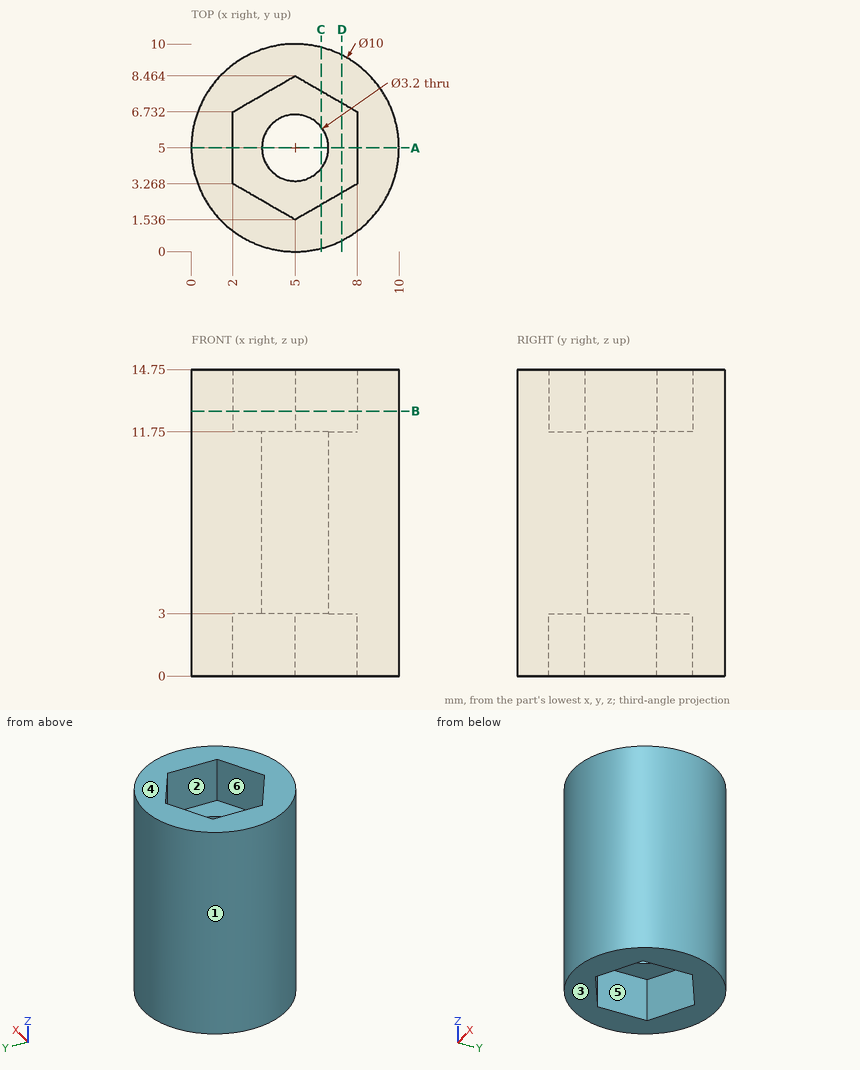
Design review of the part shown in the three views and the two pictorial views. Dimensions are in mm from the part's minimum x, y and z. A direction names the side the tool comes from. Give positions to 0.01 mm unless a question says otherwise; leave off trailing zeros. Loops run counter-clockwise (first coordinate to the right, second up) from the corner with the lowest first, then second, coordinate; pieces in that order, holes last. Notation, with made-up numbers: M 29.25,-23.5 L 81.25,-23.5 A18 cw 81.25,-8.5 Z; hole C 74,-31.75 d7. An arc over 180 degrees is marked long. Put each result on its own line as item: value. Start each with the question number.
(1) Add section C-C, the plane x = 6.25. Write out the cut boundary in (y, z), then the cut area to 3 significant figures.
(2) Add section B-B, the plane z = 12.75. Write out the cut boundary in (x, y), then the cut area to 3 significant figures.
(3) The part is to be moulded in two halves that separate along Y. For the marked faces 1, 2 and 3, say which applies: +Y half, -Y half, draft (parallel to the pull), parting line (faces both ways), or undercut.
(4) Wall thickness on L1, parallel to Y at x = 5, z = 6; L2, parallel to Z at x = 7.75, y = 6; L3, parallel to X at y = 4, z = 13.5: over which ranges is each line inside the solid? List them lowest first.
(5) Add section D-D, the plane x = 7.25. Write out the cut boundary in (y, z) (3 decimals), then the cut area to 3 significant figures.
(6) Add section A-A, the plane y = 5. Write out the cut boundary in (x, z), then the cut area to 3 significant figures.
(7) Machinability: for the marked faces 4, 5 and 6, which of the approach directions +Z, -Z, +X, -X, +Y, -Y give a long, thin tool a straight path to every point of the face, cutting with its end or side? Answer none if there is none.
(8) For pin 1 (4 mm diameter, centred on y = 8.5, z = 5, fed in from +X); pin 2 (1.5 mm diameter, centred on x = 6, z = 8, fed in from -Y), all flat-tipped, find the tip position at first contact; note any pin that passes through.
Result:
1. outline: M 0.16,0 L 2.26,0 L 2.26,3 L 4,3 L 4,11.75 L 2.26,11.75 L 2.26,14.75 L 0.16,14.75 Z; M 6,3 L 7.74,3 L 7.74,0 L 9.84,0 L 9.84,14.75 L 7.74,14.75 L 7.74,11.75 L 6,11.75 Z
1. area: 92.4 mm^2
2. outline: C 5,5 d10; hole M 2,3.27 L 5,1.54 L 8,3.27 L 8,6.73 L 5,8.46 L 2,6.73 Z
2. area: 47.4 mm^2
3. face 1: parting line
3. face 2: undercut
3. face 3: draft
4. L1: y = 0 to 3.4, 6.6 to 10
4. L2: z = 3 to 11.75
4. L3: x = 0.1 to 2, 8 to 9.9
5. outline: M 0.535,0 L 2.835,0 L 2.835,3 L 7.165,3 L 7.165,0 L 9.465,0 L 9.465,14.75 L 7.165,14.75 L 7.165,11.75 L 2.835,11.75 L 2.835,14.75 L 0.535,14.75 Z
5. area: 106 mm^2
6. outline: M 0,0 L 2,0 L 2,3 L 3.4,3 L 3.4,11.75 L 2,11.75 L 2,14.75 L 0,14.75 Z; M 6.6,3 L 8,3 L 8,0 L 10,0 L 10,14.75 L 8,14.75 L 8,11.75 L 6.6,11.75 Z
6. area: 83.5 mm^2
7. face 4: +Z, +X, -X, +Y, -Y
7. face 5: -Z
7. face 6: +Z
8. pin 1: stops at x = 9.77
8. pin 2: stops at y = 0.01
